from build123d import *

# Parameters (mm, degrees)
SKETCH1_W            = 2.54
SKETCH1_H            = 50.8
BOSS_EXTRUDE1_DEPTH  = 8.5
SKETCH2_W            = 2.54
SKETCH2_H            = 50.8
BOSS_EXTRUDE2_DEPTH  = 2.5
SKETCH3_W            = 2.54
SKETCH3_H            = 50.8
BOSS_EXTRUDE3_DEPTH  = 8.5
SKETCH4_W            = 2.54
SKETCH4_H            = 50.8
BOSS_EXTRUDE4_DEPTH  = 2.5
SKETCH5_W            = 27.94
SKETCH5_H            = 50.79
BOSS_EXTRUDE5_DEPTH  = 1.6
SKETCH6_W            = 18
SKETCH6_H            = 25.5
BOSS_EXTRUDE6_DEPTH  = 0.8
SKETCH7_W            = 15.8
SKETCH7_H            = 17.6
BOSS_EXTRUDE7_DEPTH  = 2.3
SKETCH8_W            = 7.8
SKETCH8_H            = 5.4
BOSS_EXTRUDE8_DEPTH  = 2.6
SKETCH9_W            = 3.8
SKETCH9_H            = 5.8
BOSS_EXTRUDE9_DEPTH  = 1.8
SKETCH10_W           = 3.8
SKETCH10_H           = 5.8
BOSS_EXTRUDE10_DEPTH = 1.8
SKETCH11_W           = 5.2
SKETCH11_H           = 5.2
BOSS_EXTRUDE11_DEPTH = 0.9
SKETCH12_W           = 6
SKETCH12_H           = 5
BOSS_EXTRUDE12_DEPTH = 1.6


with BuildPart() as part:
    # Sketch1 → Boss-Extrude1 (new body)
    with BuildSketch(Plane.XY.offset(10.6)):
        with Locations((-29.7, 44.42)):
            Rectangle(SKETCH1_W, SKETCH1_H)
    extrude(amount=BOSS_EXTRUDE1_DEPTH)

    # Sketch2 → Boss-Extrude2 (add)
    with BuildSketch(Plane.XY.offset(19.1)):
        with Locations((-29.7, 44.42)):
            Rectangle(SKETCH2_W, SKETCH2_H)
    extrude(amount=BOSS_EXTRUDE2_DEPTH)



with BuildPart() as body_2:
    # Sketch3 → Boss-Extrude3 (new body)
    with BuildSketch(Plane.XY.offset(10.6)):
        with Locations((-4.3, 44.42)):
            Rectangle(SKETCH3_W, SKETCH3_H)
    extrude(amount=BOSS_EXTRUDE3_DEPTH)

    # Sketch4 → Boss-Extrude4 (add)
    with BuildSketch(Plane.XY.offset(19.1)):
        with Locations((-4.3, 44.42)):
            Rectangle(SKETCH4_W, SKETCH4_H)
    extrude(amount=BOSS_EXTRUDE4_DEPTH)


with BuildPart() as part_1:
    add(part.part)

    add(body_2.part)  # Boss-Extrude5 merges body 2
    # Sketch5 → Boss-Extrude5 (add)
    with BuildSketch(Plane.XY.offset(21.6)):
        with Locations((-17, 44.425)):
            Rectangle(SKETCH5_W, SKETCH5_H)
    extrude(amount=BOSS_EXTRUDE5_DEPTH)

    # Sketch6 → Boss-Extrude6 (add)
    with BuildSketch(Plane.XY.offset(23.2)):
        with Locations((-17, 63.14)):
            Rectangle(SKETCH6_W, SKETCH6_H)
    extrude(amount=BOSS_EXTRUDE6_DEPTH)

    # Sketch7 → Boss-Extrude7 (add)
    with BuildSketch(Plane.XY.offset(24)):
        with Locations((-17, 59.89)):
            Rectangle(SKETCH7_W, SKETCH7_H)
    extrude(amount=BOSS_EXTRUDE7_DEPTH)

    # Sketch8 → Boss-Extrude8 (add)
    with BuildSketch(Plane.XY.offset(23.2)):
        with Locations((-17, 20.9)):
            Rectangle(SKETCH8_W, SKETCH8_H)
    extrude(amount=BOSS_EXTRUDE8_DEPTH)

    # Sketch9 → Boss-Extrude9 (add)
    with BuildSketch(Plane.XY.offset(23.2)):
        with Locations((-25.6, 22.7)):
            Rectangle(SKETCH9_W, SKETCH9_H)
    extrude(amount=BOSS_EXTRUDE9_DEPTH)

    # Sketch10 → Boss-Extrude10 (add)
    with BuildSketch(Plane.XY.offset(23.2)):
        with Locations((-8.4, 22.7)):
            Rectangle(SKETCH10_W, SKETCH10_H)
    extrude(amount=BOSS_EXTRUDE10_DEPTH)

    # Sketch11 → Boss-Extrude11 (add)
    with BuildSketch(Plane.XY.offset(23.2)):
        with Locations((-17, 31.1)):
            Rectangle(SKETCH11_W, SKETCH11_H)
    extrude(amount=BOSS_EXTRUDE11_DEPTH)

    # Sketch12 → Boss-Extrude12 (add)
    with BuildSketch(Plane.XY.offset(23.2)):
        with Locations((-15, 39)):
            Rectangle(SKETCH12_W, SKETCH12_H)
    extrude(amount=BOSS_EXTRUDE12_DEPTH)


solid = part_1.part
Can you work these out from the model? Positions are in its coordinate system, mm. A direction names the side the tool comes from. Coordinates: 2 decimals unless noted, no trailing zeros. Write each loop counter-clockwise with the first axis right and the second up, starting at its lowest first coordinate (ties: lowest second). Pieces come first, ordered by that corner, then holes. Notation, with made-up numbers: M -15,78 L 42,78 A22 ccw 42,105 Z; hole C 70,41.5 d1. An arc over 180 degrees is marked long. Use one line per item in the form item = value.
Q1. If we section it at D-D (y = 23): Write out the boundary of the cut face in (x, z).
Model answer:
outline = M -30.97,10.6 L -28.43,10.6 L -28.43,21.6 L -5.57,21.6 L -5.57,10.6 L -3.03,10.6 L -3.03,23.2 L -6.5,23.2 L -6.5,25 L -10.3,25 L -10.3,23.2 L -13.1,23.2 L -13.1,25.8 L -20.9,25.8 L -20.9,23.2 L -23.7,23.2 L -23.7,25 L -27.5,25 L -27.5,23.2 L -30.97,23.2 Z
Q2. I need wall thicknesses on line 1 along Y through (x, z) = (-16.75, 25); line 2 along X through (y, z) = (54.5, 21.25); line 3 along Z through (x, y) = (-8.75, 60). Which ranges of each line are inside material? Lowest first, please. Write a range as from..to.
Model answer:
line_1 = 18.2..23.6, 51.09..68.69
line_2 = -30.97..-28.43, -5.57..-3.03
line_3 = 21.6..24
Q3. If we section it at B-B (y = 33): Write out the boundary of the cut face in (x, z), then the cut area to 3 significant figures.
Model answer:
outline = M -30.97,10.6 L -28.43,10.6 L -28.43,21.6 L -5.57,21.6 L -5.57,10.6 L -3.03,10.6 L -3.03,23.2 L -14.4,23.2 L -14.4,24.1 L -19.6,24.1 L -19.6,23.2 L -30.97,23.2 Z
area = 105 mm^2
Q4. If we section it at A-A (z = 19.5): Write out the boundary of the cut face in (x, y), then the cut area to 3 significant figures.
Model answer:
outline = M -30.97,19.02 L -28.43,19.02 L -28.43,69.82 L -30.97,69.82 Z; M -5.57,19.02 L -3.03,19.02 L -3.03,69.82 L -5.57,69.82 Z
area = 258 mm^2
Q5. For P1, Ø2, axis at x = -30, z = 15.5, coming from the -Y side; P2, Ø1.8, axis at x = -20.5, y = 74.5, coming from the -Z side; P3, Ø4, axis at x = -24, y = 27, coming from the +Z side, each with a flat end and sliding along its axis, tell me the tip position at first contact or that it passes through.
Model answer:
P1 = 19.02
P2 = 23.2
P3 = 25
Q6. For faces 5 (the flat face through (-9.1, 60, 25)), 6 (the flat face through (-17, 31, 24.1)), 7 (the flat face through (-5.57, 44, 16)), which set-ups out of +Z, -Z, +X, -X, +Y, -Y let a thin tool reach every point of the face, with its end or its side?
Model answer:
face_5 = +Z, +X, +Y
face_6 = +Z, +X, -X
face_7 = -Z, +Y, -Y
Q7. We'd pull the mould along X, two halves only. Please class faces 1 (the flat face through (-6.5, 23, 24)), 2 (the flat face through (-8, 23, 25)), 3 (the flat face through (-20.9, 21, 24)), 4 (the flat face through (-28.43, 44, 16)): +X half, -X half, draft (parallel to the pull), parting line (faces both ways), or undercut.
Model answer:
face_1 = +X half
face_2 = draft
face_3 = undercut
face_4 = undercut
